Source: CAD feature listing. Evaluate the final solid. Frame: model axes, mm. A direction names the side the tool comes from. Give positions to 0.01 mm unless a question says otherwise; leave off trailing zeros. Write each loop counter-clockwise with the first axis right and the second up, starting at its lowest first coordinate (ties: lowest second). Pieces come first, ordered by that corner, then holes. Notation, with made-up numbers: M 52.5,48 L 60.5,48 A16 cw 60.5,57 Z; hole C -8,74 d2. An arc over 180 degrees is marked long. Return JSON: item names as keys, results as strings.
```python
from build123d import *

# Parameters (mm, degrees)
SKETCH1_W                 = 279.4
SKETCH1_H                 = 101.6
BOSS_EXTRUDE1_DEPTH       = 6.35
SKETCH2_R                 = 13.97
BOSS_EXTRUDE3_DEPTH       = 5.55625
SKETCH9_R                 = 11.1125
CUT_EXTRUDE4_DEPTH        = 4.445
CUT_EXTRUDE5_START        = -5.55625
SKETCH10_R                = 11.1125
CUT_EXTRUDE5_DEPTH        = 5.55625
SKETCH11_R                = 7.9375
CUT_EXTRUDE6_DEPTH        = 285.078633923
SKETCH12_R                = 6.35
CUT_EXTRUDE7_DEPTH        = 285.051619429
SKETCH22_W                = 63.5
SKETCH22_H                = 63.5
BOSS_EXTRUDE7_DEPTH       = 12.7
SKETCH25_W                = 50.8
SKETCH25_H                = 50.8
CUT_EXTRUDE11_DEPTH       = 15.875
SKETCH32_R                = 4.7625
CUT_EXTRUDE12_DEPTH       = 6.35
SKETCH38_W                = 46.99
SKETCH38_H                = 18.470251096
CUT_EXTRUDE13_DEPTH       = 6.35
SKETCH60_R                = 4.7625
CUT_EXTRUDE23_DEPTH       = 6.35
SKETCH64_R                = 4.7625
CUT_EXTRUDE24_DEPTH       = 285.264471927
SKETCH69_W                = 33.02
SKETCH69_H                = 6.35
BOSS_EXTRUDE10_DEPTH      = 19.05
SKETCH70_R                = 4.7625
SKETCH70_R_2              = 2.54
CUT_EXTRUDE26_DEPTH       = 6.35
SKETCH76_R                = 4.7625
CUT_EXTRUDE29_DEPTH       = 6.35
SKETCH77_W                = 46.99
SKETCH77_H                = 16.7871648
CUT_EXTRUDE30_DEPTH       = 6.35
SKETCH78_W                = 49.276
SKETCH78_H                = 66.342584104
CUT_EXTRUDE32_DEPTH       = 1.524
SKETCH79_R                = 4.7625
CUT_EXTRUDE33_DEPTH       = 4.826
CUT_EXTRUDE34_START       = -3.175
CUT_EXTRUDE34_OUTLINE_R   = 4.7625
CUT_EXTRUDE34_OUTLINE_R_2 = 7.9375
CUT_EXTRUDE34_DEPTH       = 19.05


# Read off the part's stored shape, not the designer's step: Cut-Extrude34
with BuildPart() as part:
    # Sketch1 → Boss-Extrude1 (new body)
    with BuildSketch(Plane(origin=(0, 0, 0), x_dir=(1, 0, 0), z_dir=(0, 1, 0))):
        with Locations((-139.7, 0)):
            Rectangle(SKETCH1_W, SKETCH1_H)
    extrude(amount=BOSS_EXTRUDE1_DEPTH)

    # Sketch2 → Boss-Extrude3 (add)
    with BuildSketch(Plane(origin=(0, 6.35, 0), x_dir=(1, 0, 0), z_dir=(0, 1, 0))):
        with Locations(Location((-258.510557857, 0, 0), (0, 0, 90))):
            Circle(SKETCH2_R)
    extrude(amount=BOSS_EXTRUDE3_DEPTH)

    # Sketch9 → Cut-Extrude4 (cut)
    with BuildSketch(Plane(origin=(0, 11.90625, 0), x_dir=(1, 0, 0), z_dir=(0, 1, 0))):
        with Locations(Location((-258.510557857, 0, 0), (0, 0, 270))):
            Circle(SKETCH9_R)
    extrude(amount=-CUT_EXTRUDE4_DEPTH, mode=Mode.SUBTRACT)

    # Sketch10 → Cut-Extrude5 (cut)
    with BuildSketch(Plane(origin=(0, 0, 0), x_dir=(-1, 0, 0), z_dir=(0, -1, 0)).offset(CUT_EXTRUDE5_START)):
        with Locations(Location((258.510557857, 0, 0), (0, 0, 270))):
            Circle(SKETCH10_R)
    extrude(amount=CUT_EXTRUDE5_DEPTH, mode=Mode.SUBTRACT)

    # Sketch11 → Cut-Extrude6 (cut, through all)
    with BuildSketch(Plane(origin=(0, 7.46125, 0), x_dir=(1, 0, 0), z_dir=(0, 1, 0))):
        with Locations(Location((-258.510557857, 0, 0), (0, 0, 270))):
            Circle(SKETCH11_R)
    extrude(amount=-CUT_EXTRUDE6_DEPTH, mode=Mode.SUBTRACT)

    # Sketch12 → Cut-Extrude7 (cut, through all)
    with BuildSketch(Plane(origin=(0, 6.35, 0), x_dir=(1, 0, 0), z_dir=(0, 1, 0))):
        with Locations(Location((-134.666203771, 0, 0), (0, 0, 270))):
            Circle(SKETCH12_R)
    extrude(amount=-CUT_EXTRUDE7_DEPTH, mode=Mode.SUBTRACT)

    # Sketch22 → Boss-Extrude7 (add)
    with BuildSketch(Plane(origin=(0, 6.35, 0), x_dir=(1, 0, 0), z_dir=(0, 1, 0))):
        with Locations((-134.666203771, 0)):
            Rectangle(SKETCH22_W, SKETCH22_H)
    extrude(amount=BOSS_EXTRUDE7_DEPTH)

    # Sketch25 → Cut-Extrude11 (cut)
    with BuildSketch(Plane(origin=(0, 19.05, 0), x_dir=(1, 0, 0), z_dir=(0, 1, 0))):
        with Locations((-134.666203771, 0)):
            Rectangle(SKETCH25_W, SKETCH25_H)
    extrude(amount=-CUT_EXTRUDE11_DEPTH, mode=Mode.SUBTRACT)

    # Sketch32 → Cut-Extrude12 (cut)
    with BuildSketch(Plane(origin=(0, 6.35, 0), x_dir=(1, 0, 0), z_dir=(0, 1, 0))):
        with Locations(Location((-67.44195898, -40.64, 0), (0, 0, 270))):
            Circle(SKETCH32_R)
        with Locations(Location((-81.41195898, -40.64, 0), (0, 0, 270))):
            Circle(SKETCH32_R)
        with Locations(Location((-67.44195898, 40.64, 0), (0, 0, 270))):
            Circle(SKETCH32_R)
        with Locations(Location((-81.41195898, 40.64, 0), (0, 0, 270))):
            Circle(SKETCH32_R)
    extrude(amount=-CUT_EXTRUDE12_DEPTH, mode=Mode.SUBTRACT)

    # Sketch38 → Cut-Extrude13 (cut)
    with BuildSketch(Plane(origin=(0, 6.35, 0), x_dir=(1, 0, 0), z_dir=(0, 1, 0))):
        with Locations((-23.495, -24.777709652)):
            Rectangle(SKETCH38_W, SKETCH38_H)
    extrude(amount=-CUT_EXTRUDE13_DEPTH, mode=Mode.SUBTRACT)

    # Sketch60 → Cut-Extrude23 (cut)
    with BuildSketch(Plane(origin=(0, 6.35, 0), x_dir=(1, 0, 0), z_dir=(0, 1, 0))):
        with Locations(Location((-231.7492444, 41.324145444, 0), (0, 0, 270))):
            Circle(SKETCH60_R)
        with Locations(Location((-231.7492444, -39.369341378, 0), (0, 0, 270))):
            Circle(SKETCH60_R)
        with Locations(Location((-173.509244294, -39.369341378, 0), (0, 0, 270))):
            Circle(SKETCH60_R)
        with Locations(Location((-173.509244294, 41.324145444, 0), (0, 0, 270))):
            Circle(SKETCH60_R)
    extrude(amount=-CUT_EXTRUDE23_DEPTH, mode=Mode.SUBTRACT)

    # Sketch64 → Cut-Extrude24 (cut, through all)
    with BuildSketch(Plane(origin=(0, 6.35, 0), x_dir=(1, 0, 0), z_dir=(0, 1, 0))):
        with Locations(Location((-145.334203771, -41.275, 0), (0, 0, 270))):
            Circle(SKETCH64_R)
        with Locations(Location((-123.998203771, -41.275, 0), (0, 0, 270))):
            Circle(SKETCH64_R)
    cut_extrude24 = extrude(amount=-CUT_EXTRUDE24_DEPTH, mode=Mode.SUBTRACT)

    # Mirror1: Cut-Extrude24 across plane
    add(cut_extrude24.mirror(Plane.XY), mode=Mode.SUBTRACT)

    # Sketch69 → Boss-Extrude10 (add)
    with BuildSketch(Plane.XY.offset(50.8)):
        with Locations((-70.465355554, 3.175)):
            Rectangle(SKETCH69_W, SKETCH69_H)
    boss_extrude10 = extrude(amount=BOSS_EXTRUDE10_DEPTH)

    # Sketch70 → Cut-Extrude26 (cut)
    with BuildSketch(Plane(origin=(0, 6.35, 0), x_dir=(1, 0, 0), z_dir=(0, 1, 0))):
        with Locations(Location((-76.815355554, -60.325, 0), (0, 0, 270))):
            Circle(SKETCH70_R)
        with Locations(Location((-64.115355554, -60.325, 0), (0, 0, 270))):
            Circle(SKETCH70_R_2)
    cut_extrude26 = extrude(amount=-CUT_EXTRUDE26_DEPTH, mode=Mode.SUBTRACT)

    # Mirror2: Boss-Extrude10, Cut-Extrude26 across plane
    add(boss_extrude10.mirror(Plane.XY))
    add(cut_extrude26.mirror(Plane.XY), mode=Mode.SUBTRACT)

    # Sketch76 → Cut-Extrude29 (cut)
    with BuildSketch(Plane(origin=(0, 6.35, 0), x_dir=(1, 0, 0), z_dir=(0, 1, 0))):
        with Locations(Location((-264.668, 24.13, 0), (0, 0, 270))):
            Circle(SKETCH76_R)
        with Locations(Location((-252.222, 24.13, 0), (0, 0, 270))):
            Circle(SKETCH76_R)
    extrude(amount=-CUT_EXTRUDE29_DEPTH, mode=Mode.SUBTRACT)

    # Sketch77 → Cut-Extrude30 (cut)
    with BuildSketch(Plane(origin=(0, 6.35, 0), x_dir=(1, 0, 0), z_dir=(0, 1, 0))):
        with Locations((-23.495, -42.4064176)):
            Rectangle(SKETCH77_W, SKETCH77_H)
    extrude(amount=-CUT_EXTRUDE30_DEPTH, mode=Mode.SUBTRACT)

    # Sketch78 → Cut-Extrude32 (cut)
    with BuildSketch(Plane(origin=(0, 6.35, 0), x_dir=(1, 0, 0), z_dir=(0, 1, 0))):
        with Locations((-24.638, 17.628707948)):
            Rectangle(SKETCH78_W, SKETCH78_H)
    extrude(amount=-CUT_EXTRUDE32_DEPTH, mode=Mode.SUBTRACT)

    # Sketch79 → Cut-Extrude33 (cut)
    with BuildSketch(Plane(origin=(0, 4.826, 0), x_dir=(1, 0, 0), z_dir=(0, 1, 0))):
        with Locations(Location((-23.876, 15.191415896, 0), (0, 0, 270))):
            Circle(SKETCH79_R)
    extrude(amount=-CUT_EXTRUDE33_DEPTH, mode=Mode.SUBTRACT)

    # Cut-Extrude34 outline → Cut-Extrude34 (cut)
    with BuildSketch(Plane(origin=(0, 3.175, 0), x_dir=(1, 0, 0), z_dir=(0, 1, 0)).offset(CUT_EXTRUDE34_START)):
        with BuildLine():
            ThreePointArc((-134.666203771, -6.35), (-141.016203771, 0), (-134.666203771, 6.35))
            Line((-134.666203771, 6.35), (-134.666203771, 50.8))
            Line((-134.666203771, 50.8), (-279.4, 50.8))
            Line((-279.4, 50.8), (-279.4, -50.8))
            Line((-279.4, -50.8), (-134.666203771, -50.8))
            Line((-134.666203771, -50.8), (-134.666203771, -6.35))
        make_face()
        with Locations((-231.7492444, 41.324145444)):
            Circle(CUT_EXTRUDE34_OUTLINE_R, mode=Mode.SUBTRACT)
        with Locations((-173.509244294, 41.324145444)):
            Circle(CUT_EXTRUDE34_OUTLINE_R, mode=Mode.SUBTRACT)
        with Locations((-145.334203771, 41.275)):
            Circle(CUT_EXTRUDE34_OUTLINE_R, mode=Mode.SUBTRACT)
        with Locations((-231.7492444, -39.369341378)):
            Circle(CUT_EXTRUDE34_OUTLINE_R, mode=Mode.SUBTRACT)
        with Locations((-173.509244294, -39.369341378)):
            Circle(CUT_EXTRUDE34_OUTLINE_R, mode=Mode.SUBTRACT)
        with Locations((-145.334203771, -41.275)):
            Circle(CUT_EXTRUDE34_OUTLINE_R, mode=Mode.SUBTRACT)
        with Locations((-264.668, 24.13)):
            Circle(CUT_EXTRUDE34_OUTLINE_R, mode=Mode.SUBTRACT)
        with Locations((-252.222, 24.13)):
            Circle(CUT_EXTRUDE34_OUTLINE_R, mode=Mode.SUBTRACT)
        with Locations((-258.510557857, 0)):
            Circle(CUT_EXTRUDE34_OUTLINE_R_2, mode=Mode.SUBTRACT)
    extrude(amount=CUT_EXTRUDE34_DEPTH, mode=Mode.SUBTRACT)


solid = part.part
```
1) Cut plane A-A, the plane x = -104.5. Return the cut outline in (y, z).
Numbers:
{"outline": "M 0,-50.8 L 6.35,-50.8 L 6.35,-31.75 L 19.05,-31.75 L 19.05,31.75 L 6.35,31.75 L 6.35,50.8 L 0,50.8 Z"}
2) Cut plane D-D, the plane x = -74. Return the cut outline in (y, z).
Numbers:
{"outline": "M 0,-69.85 L 6.35,-69.85 L 6.35,-64.17 L 0,-64.17 Z; M 0,-56.48 L 6.35,-56.48 L 6.35,56.48 L 0,56.48 Z; M 0,64.17 L 6.35,64.17 L 6.35,69.85 L 0,69.85 Z"}
3) Cut plane B-B, the plane z = 40.64. Return the cut outline in (x, y), then the cut area to 3 significant figures.
Numbers:
{"outline": "M -134.67,0 L -128.72,0 L -128.72,6.35 L -134.67,6.35 Z; M -119.28,0 L -86.17,0 L -86.17,6.35 L -119.28,6.35 Z; M -76.65,0 L -72.2,0 L -72.2,6.35 L -76.65,6.35 Z; M -62.68,0 L -46.99,0 L -46.99,6.35 L -62.68,6.35 Z", "area": "376 mm²"}
4) Set-up query: faces 4 (the face through (-46.99, 3, 33)), 5 (the face through (-27, 2, -50.8)), 6 (the face through (-122, 11, -25.4)), 7 (the face through (-111, 3, -50.8)). Return all of +Z, -Z, +X, -X, +Y, -Y with unobstructed straight access to the full face (end or side cutting, diameter ignored); none if empty.
Numbers:
{"face 4": "+Z, +X, +Y, -Y", "face 5": "-Z, +X, +Y, -Y", "face 6": "-X, +Y", "face 7": "-Z, -X, +Y, -Y"}
5) Cut plane C-C, the plane y = 13.5. Return the cut outline in (x, z), then the cut area to 3 significant figures.
Numbers:
{"outline": "M -134.67,-31.75 L -102.92,-31.75 L -102.92,31.75 L -134.67,31.75 L -134.67,25.4 L -109.27,25.4 L -109.27,-25.4 L -134.67,-25.4 Z", "area": "726 mm²"}
6) Draft query along Z for faces 1 (the face through (-68, 0, -1)), 2 (the face through (-119, 13, 31.75)), 3 (the face through (-128.318, 1.61, 0.14)). Return one class per face: released by +Z, released by -Z, zero draft, split by the parting line, or undercut.
Numbers:
{"face 1": "zero draft", "face 2": "released by +Z", "face 3": "undercut"}
7) Contact query for flat-ended pins moving along their axis: pin 1 Ø1.9 at (y, z) = (2, -58.5) entering from -X; pin 2 Ø11 at (x, z) = (-76.82, -60.32) entering from +Y; pin 3 Ø6.5 at (x, y) = (-122, 11.5) entering from +Z; pin 4 Ø7.5 at (x, z) = (-124, -41.28) entering from -Y. Output: stop coordinate, or through.
Numbers:
{"pin 1": "stops at x = -86.98", "pin 2": "stops at y = 6.35", "pin 3": "stops at z = 31.75", "pin 4": "passes through"}
8) Line query: line 1 (Z direction, x = -82, y = 4.5); line 2 (Z direction, x = -127, y = 8); line 3 (Z direction, x = -78, y = 6.25). Output: solid intervals per line, ascending. Write a range as [from, to].
Numbers:
{"line 1": "z = [-69.85, -45.37], [-35.91, 35.91], [45.37, 69.85]", "line 2": "z = [-31.75, -25.4], [25.4, 31.75]", "line 3": "z = [-69.85, -64.94], [-55.71, -43.96], [-37.32, 37.32], [43.96, 55.71], [64.94, 69.85]"}
